from build123d import *

# Parameters (mm, degrees)
F1_DEPTH     = 3
F0_W         = 29.5
F0_H         = 29.5
F2_DEPTH     = 14.5
F3_DEPTH     = 3
F4_DEPTH     = 1.5
F6_W         = 12
F6_H         = 2
F7_DEPTH     = 1
F8_SIZE2     = 1.99999
F8_SIZE      = 0.99999
F9_W         = 1.2
F9_H         = 2
F10_DEPTH    = 1
F11_SIZE2    = 1.99999
F11_SIZE     = 0.99999
F12_SIZE2    = 1.99999
F12_SIZE     = 0.99999
F13_T1_DEPTH = 45.958771123
F13_T3_DEPTH = 45.958771123
F5_R         = 1.35
F14_DEPTH    = 30
F15_SIZE     = 2


# Not quite as in the source:
# - a fillet or chamfer that OpenCascade refuses, or shapes differently, is made with other operations: its cross-section is extruded or revolved along the edge and cut away or added
# - a fillet or chamfer is up to 0.001 mm smaller than in the source, because OpenCascade refuses the exact size


with BuildPart() as f1:
    # F0 (on Top) → F1 (new body)
    with BuildSketch(Plane.XY):
        with BuildLine():
            ThreePointArc((12.75, 11), (9.7625631329, 9.7625631329), (11, 12.75))
            Line((11, 12.75), (-11, 12.75))
            ThreePointArc((-11, 12.75), (-9.7625631329, 12.2374368671), (-9.25, 11))
            ThreePointArc((-9.25, 11), (-11, 9.25), (-12.75, 11))
            Line((-12.75, 11), (-12.75, -5e-10))
            ThreePointArc((-12.75, -5e-10), (-11.9445436484, 1.9445436481), (-10, 2.75))
            Line((-10, 2.75), (-8.75, 2.75))
            Line((-8.75, 2.75), (-8.75, 8.75))
            Line((-8.75, 8.75), (8.75, 8.75))
            Line((8.75, 8.75), (8.75, 2.75))
            Line((8.75, 2.75), (10, 2.75))
            ThreePointArc((10, 2.75), (11.9445436484, 1.9445436481), (12.75, -5e-10))
            Line((12.75, -5e-10), (12.75, 11))
        make_face()
        with BuildLine():
            ThreePointArc((-12.75, 11), (-12.2374368671, 12.2374368671), (-11, 12.75))
            Line((-11, 12.75), (-12.75, 12.75))
            Line((-12.75, 12.75), (-12.75, 11))
        make_face()
        with BuildLine():
            Line((12.75, 11), (12.75, 12.75))
            Line((12.75, 12.75), (11, 12.75))
            ThreePointArc((11, 12.75), (12.2374368671, 12.2374368671), (12.75, 11))
        make_face()
        with BuildLine():
            ThreePointArc((12.75, 11), (12.2374368671, 12.2374368671), (11, 12.75))
            ThreePointArc((11, 12.75), (9.7625631329, 9.7625631329), (12.75, 11))
        make_face()
        with BuildLine():
            ThreePointArc((-9.25, 11), (-9.7625631329, 12.2374368671), (-11, 12.75))
            ThreePointArc((-11, 12.75), (-12.2374368671, 12.2374368671), (-12.75, 11))
            ThreePointArc((-12.75, 11), (-11, 9.25), (-9.25, 11))
        make_face()
    extrude(amount=F1_DEPTH)



with BuildPart() as f1b:
    # F0 (on Top) → F1, piece 2 (new body)
    with BuildSketch(Plane.XY):
        with BuildLine():
            Line((12.75, -11), (12.75, -5e-10))
            ThreePointArc((12.75, -5e-10), (11.9445436481, -1.9445436484), (10, -2.75))
            Line((10, -2.75), (8.75, -2.75))
            Line((8.75, -2.75), (8.75, -8.75))
            Line((8.75, -8.75), (-8.75, -8.75))
            Line((-8.75, -8.75), (-8.75, -2.75))
            Line((-8.75, -2.75), (-10, -2.75))
            ThreePointArc((-10, -2.75), (-11.9445436481, -1.9445436484), (-12.75, -5e-10))
            Line((-12.75, -5e-10), (-12.75, -11))
            ThreePointArc((-12.75, -11), (-11, -9.25), (-9.25, -11))
            ThreePointArc((-9.25, -11), (-9.7625631329, -12.2374368671), (-11, -12.75))
            Line((-11, -12.75), (11, -12.75))
            ThreePointArc((11, -12.75), (9.7625631329, -9.7625631329), (12.75, -11))
        make_face()
        with BuildLine():
            ThreePointArc((-11, -12.75), (-12.2374368671, -12.2374368671), (-12.75, -11))
            Line((-12.75, -11), (-12.75, -12.75))
            Line((-12.75, -12.75), (-11, -12.75))
        make_face()
        with BuildLine():
            Line((12.75, -12.75), (12.75, -11))
            ThreePointArc((12.75, -11), (12.2374368671, -12.2374368671), (11, -12.75))
            Line((11, -12.75), (12.75, -12.75))
        make_face()
        with BuildLine():
            ThreePointArc((11, -12.75), (12.2374368671, -12.2374368671), (12.75, -11))
            ThreePointArc((12.75, -11), (9.7625631329, -9.7625631329), (11, -12.75))
        make_face()
        with BuildLine():
            ThreePointArc((-9.25, -11), (-11, -9.25), (-12.75, -11))
            ThreePointArc((-12.75, -11), (-12.2374368671, -12.2374368671), (-11, -12.75))
            ThreePointArc((-11, -12.75), (-9.7625631329, -12.2374368671), (-9.25, -11))
        make_face()
    extrude(amount=F1_DEPTH)


with BuildPart() as f1_1:
    add(f1.part)

    add(f1b.part)  # F2 merges F1b
    # F0 (on Top) → F2 (join)
    with BuildSketch(Plane.XY):
        Rectangle(F0_W, F0_H)
        Polygon((11, 12.75), (12.75, 12.75), (12.75, 11), (12.75, -5e-10), (12.75, -11), (12.75, -12.75), (11, -12.75), (-11, -12.75), (-12.75, -12.75), (-12.75, -11), (-12.75, -5e-10), (-12.75, 11), (-12.75, 12.75), (-11, 12.75), align=None, mode=Mode.SUBTRACT)
    extrude(amount=F2_DEPTH)

    # F0 (on Top) → F3 (cut)
    with BuildSketch(Plane.XY):
        with BuildLine():
            ThreePointArc((-9.25, 11), (-9.7625631329, 12.2374368671), (-11, 12.75))
            ThreePointArc((-11, 12.75), (-12.2374368671, 12.2374368671), (-12.75, 11))
            ThreePointArc((-12.75, 11), (-11, 9.25), (-9.25, 11))
        make_face()
        with BuildLine():
            ThreePointArc((12.75, 11), (12.2374368671, 12.2374368671), (11, 12.75))
            ThreePointArc((11, 12.75), (9.7625631329, 9.7625631329), (12.75, 11))
        make_face()
        with BuildLine():
            ThreePointArc((-9.25, -11), (-11, -9.25), (-12.75, -11))
            ThreePointArc((-12.75, -11), (-12.2374368671, -12.2374368671), (-11, -12.75))
            ThreePointArc((-11, -12.75), (-9.7625631329, -12.2374368671), (-9.25, -11))
        make_face()
        with BuildLine():
            ThreePointArc((11, -12.75), (12.2374368671, -12.2374368671), (12.75, -11))
            ThreePointArc((12.75, -11), (9.7625631329, -9.7625631329), (11, -12.75))
        make_face()
    extrude(amount=F3_DEPTH, mode=Mode.SUBTRACT)

    # F0 (on Top) → F4 (join)
    with BuildSketch(Plane.XY):
        with BuildLine():
            ThreePointArc((12.75, 11), (12.2374368671, 12.2374368671), (11, 12.75))
            ThreePointArc((11, 12.75), (9.7625631329, 9.7625631329), (12.75, 11))
        make_face()
        with BuildLine():
            ThreePointArc((-9.25, 11), (-9.7625631329, 12.2374368671), (-11, 12.75))
            ThreePointArc((-11, 12.75), (-12.2374368671, 12.2374368671), (-12.75, 11))
            ThreePointArc((-12.75, 11), (-11, 9.25), (-9.25, 11))
        make_face()
        with BuildLine():
            ThreePointArc((-9.25, -11), (-11, -9.25), (-12.75, -11))
            ThreePointArc((-12.75, -11), (-12.2374368671, -12.2374368671), (-11, -12.75))
            ThreePointArc((-11, -12.75), (-9.7625631329, -12.2374368671), (-9.25, -11))
        make_face()
        with BuildLine():
            ThreePointArc((11, -12.75), (12.2374368671, -12.2374368671), (12.75, -11))
            ThreePointArc((12.75, -11), (9.7625631329, -9.7625631329), (11, -12.75))
        make_face()
    extrude(amount=F4_DEPTH)

    # F6 (on face) → F7 (join)
    with BuildSketch(Plane.XZ.offset(-12.75)):
        with Locations((2.75, 11.3)):
            Rectangle(F6_W, F6_H)
    extrude(amount=F7_DEPTH)

    # F8 (size 1 and 2 in the source; OpenCascade refuses exactly that, so slightly less here)
    f8_edges = [f1_1.edges().sort_by_distance(p)[0] for p in [
        (2.75, 11.75, 12.3),
    ]]
    f8_side = f1_1.faces().sort_by_distance((2.75, 12.25, 12.3))[0]
    chamfer(f8_edges, length=F8_SIZE, length2=F8_SIZE2, reference=f8_side)

    # F9 (on face) → F10 (join)
    with BuildSketch(Plane(origin=(0, -12.75, 0), x_dir=(-1, 0, 0), z_dir=(0, 1, 0))):
        with Locations((-8.85, 11.3)):
            Rectangle(F9_W, F9_H)
        with Locations((8.85, 11.3)):
            Rectangle(F9_W, F9_H)
    extrude(amount=F10_DEPTH)

    # F11 (size 1 and 2 in the source; OpenCascade refuses exactly that, so slightly less here)
    f11_edges = [f1_1.edges().sort_by_distance(p)[0] for p in [
        (8.85, -11.75, 12.3),
    ]]
    f11_side = f1_1.faces().sort_by_distance((8.85, -12.25, 12.3))[0]
    chamfer(f11_edges, length=F11_SIZE, length2=F11_SIZE2, reference=f11_side)

    # F12 (size 1 and 2 in the source; OpenCascade refuses exactly that, so slightly less here)
    f12_edges = [f1_1.edges().sort_by_distance(p)[0] for p in [
        (-8.85, -11.75, 12.3),
    ]]
    f12_side = f1_1.faces().sort_by_distance((-8.85, -12.25, 12.3))[0]
    chamfer(f12_edges, length=F12_SIZE, length2=F12_SIZE2, reference=f12_side)

    # F13: chamfer of 3.2 on 4 edges, made by hand

    # F13_s2 → F13_t1 (cut)
    with BuildSketch(Plane.YZ.offset(-22.9793855615)):
        Polygon((14.75, 3.2), (11.55, 0), (14.75, 0), align=None)
        Polygon((-14.75, 3.2), (-11.55, 0), (-14.75, 0), align=None)
    extrude(amount=F13_T1_DEPTH, mode=Mode.SUBTRACT)

    # F13_s4 → F13_t3 (cut)
    with BuildSketch(Plane.XZ.offset(-22.9793855615)):
        Polygon((-14.75, 3.2), (-11.55, 0), (-14.75, 0), align=None)
        Polygon((14.75, 3.2), (11.55, 0), (14.75, 0), align=None)
    extrude(amount=F13_T3_DEPTH, mode=Mode.SUBTRACT)

    # F5 (on face) → F14 (cut)
    with BuildSketch(Plane(origin=(-14.75, 0, 0), x_dir=(0, -1, 0), z_dir=(-1, 0, 0))):
        with Locations((4.75, 12)):
            Circle(F5_R)
        with Locations((-3.75, 12)):
            Circle(F5_R)
    extrude(amount=-F14_DEPTH, mode=Mode.SUBTRACT)

    # F15
    f15_edges = [f1_1.edges().sort_by_distance(p)[0] for p in [
        (14.75, 14.75, 8.85),
        (-14.75, 14.75, 8.85),
        (14.75, -14.75, 8.85),
        (-14.75, -14.75, 8.85),
    ]]
    chamfer(f15_edges, length=F15_SIZE)


solid = f1_1.part
Could you check a few things on this model? Use its own coordinates, in mm. A direction names the side the tool comes from. Coordinates: 2 decimals unless noted, no trailing zeros. Order: outer loops, then holes, each group sorted by start corner. A loop starts at its lowest first (then second) coordinate and runs counter-clockwise, first axis right, second up. Notation, with made-up numbers: (27.25, 68.5) - (64.25, 68.5) arc R23 ccw to (64.25, 96.5) - close; hole circle Ø5 at (9.25, 80). An arc over 180 degrees is marked (long way). Answer in a Markdown table with one row per item. Add a question column.
(1) If we mould it in two halves opening along Y, with no side actions, what happens to faces 5 (the face through (13, 0, 14.5)), 6 (the face through (13.8, -13.7, 8.3)), 7 (the face through (2.666, 12.243, 11.286))? For each: released by +Y, released by -Y, zero draft, split by the parting line, or undercut.
(2) On a 3-axis mill with a long thin cutter (end or side, diameter ignored), from which of +Z, -Z, +X, -X, +Y, -Y can I reach the whole of each face in a straight line? I mean faces 1 (the face through (3, 12, 10.3)), 2 (the face through (-13.7, -13.8, 8.3)), 3 (the face through (-12.4, -12.3, 3)), 4 (the face through (-9, 2.75, 1)). Say none if no direction works.
(3) I need wall thicknesses on L1, parallel to X at y = -1, z = 6; L2, parallel to X at y = -11, z = 2.35. Which ranges of each line are inside material? Lowest first, please.
(4) If we section it at C-C, the plane x = -4: Please give me the cut outline in (y, z).
(5) Will these pins go through, and if not, where does the flat tip stop? pin 1 (1 mm diameter, centred on x = 9, y = 2.5, fed in from -Z); pin 2 (6.5 mm diameter, centred on x = -6, y = -8, fed in from +Z); pin 3 (1.4 mm diameter, centred on x = 9.5, z = 1.5, fed in from +Y); pin 4 (0.9 mm diameter, centred on y = 6.5, z = 1.5, fed in from -X).
(6) If we section it at B-B, the plane z = 6.5: Please give me the cut outline in (x, y), then the cut area to 3 significant figures.
(7) If we section it at A-A, the plane y = -4.75: Please give me the cut outline in (x, z).
Results are:
| question | item | result |
|---|---|---|
| 1 | face 5 | zero draft |
| 1 | face 6 | released by -Y |
| 1 | face 7 | undercut |
| 2 | face 1 | none |
| 2 | face 2 | +Z, -Z, -X, -Y |
| 2 | face 3 | +Z |
| 2 | face 4 | +Z, -Z |
| 3 | L1 | x = -14.75 to -12.75, 12.75 to 14.75 |
| 3 | L2 | x = -13.9 to -12.75, -9.25 to 9.25, 12.75 to 13.9 |
| 4 | outline | (-14.75, 3.2) - (-11.55, 0) - (-8.75, 0) - (-8.75, 3) - (-12.75, 3) - (-12.75, 14.5) - (-14.75, 14.5) - close; (8.75, 0) - (11.55, 0) - (14.75, 3.2) - (14.75, 14.5) - (12.75, 14.5) - (12.75, 3) - (8.75, 3) - close |
| 5 | pin 1 | stops at z = 0 |
| 5 | pin 2 | stops at z = 3 |
| 5 | pin 3 | stops at y = 13.75 |
| 5 | pin 4 | stops at x = -13.5 |
| 6 | outline | (-14.75, -12.75) - (-12.75, -14.75) - (12.75, -14.75) - (14.75, -12.75) - (14.75, 12.75) - (12.75, 14.75) - (-12.75, 14.75) - (-14.75, 12.75) - close; hole (-12.75, -12.75) - (12.75, -12.75) - (12.75, 12.75) - (-12.75, 12.75) - close |
| 6 | area | 212 mm2 |
| 7 | outline | (-14.75, 3.2) - (-11.55, 0) - (-8.75, 0) - (-8.75, 3) - (-12.75, 3) - (-12.75, 10.65) - (-14.75, 10.65) - close; (-14.75, 13.35) - (-12.75, 13.35) - (-12.75, 14.5) - (-14.75, 14.5) - close; (8.75, 0) - (11.55, 0) - (14.75, 3.2) - (14.75, 10.65) - (12.75, 10.65) - (12.75, 3) - (8.75, 3) - close; (12.75, 13.35) - (14.75, 13.35) - (14.75, 14.5) - (12.75, 14.5) - close |
